Autodesk Inventor part; units mm, degrees
ref_plane "YZ Plane" through (0, 0, 0) normal (1, 0, 0) x (0, 1, 0)
ref_plane "XZ Plane" through (0, 0, 0) normal (0, 1, 0) x (-1, 0, 0)
ref_plane "XY Plane" through (0, 0, 0) normal (0, 0, 1) x (1, 0, 0)
sketch "Sketch2" plane through (0, 0, 0) normal (0, 0, 1) x (1, 0, 0)
  line L0 (0, 0) -> (48.55, 0)
  line L1 (48.55, 0) -> (48.55, -13)
  line L2 (48.55, -13) -> (44.55, -13)
  line L3 (44.55, -13) -> (44.55, -4)
  line L4 (44.55, -4) -> (38.45, -4)
  line L5 (38.45, -4) -> (38.45, -7)
  line L6 (38.45, -7) -> (0, -7)
  line L7 (0, -7) -> (0, 0)
  dimension "d0" = 48.55
  dimension "d1" = 4
  dimension "d2" = 6.1
  dimension "d3" = 13
  dimension "d4" = 4
  dimension "d5" = 7
revolve "Revolution1" add sketch "Sketch2" angle 360 about axis through (0, -7, 0) along (0, 1, 0)
fillet "Fillet1" radius 3 1 edges at (-48.55, 0, 0)
sketch "Sketch3" plane through (0, -7, 0) normal (0, -1, 0) x (1, 0, 0)
  circle A0 centre (0, -19.85) radius 17
  circle A1 centre (0, 0) radius 38.45
  circle A2 centre (17.1906, 9.925) radius 17
  circle A3 centre (-17.1906, 9.925) radius 17
  dimension "d8" = 34
  dimension "d11" = 360
  dimension "d15" = 19.85
extrude "Extrusion1" cut sketch "Sketch3" against normal blind 5.5 contours A0 | A2 | A3
sketch "Sketch5" plane through (0, -7, 0) normal (0, -1, 0) x (1, 0, 0)
  circle A0 centre (-25.9808, -15) radius 6.25
  line L0 (-25.9808, -15) -> (0, 0) construction
  line L1 (0, 0) -> (-9.9215, 0) construction
  dimension "d16" = 12.5
  dimension "d17" = 30
  dimension "d20" = 30
extrude "Extrusion2" cut sketch "Sketch5" against normal through all
properties part number "lid-proto-v2"
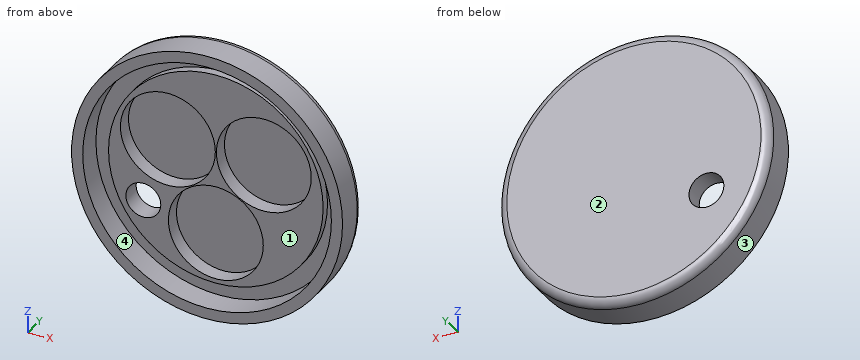
The listing builds one solid part. Answer for the finished solid, in the listing's coordinates (mm). Face numbers are marked on the shaded views. Coordinates: 2 decimals unless noted, no trailing zeros. Write each loop counter-clockwise with the first axis right and the second up, starting at its lowest first coordinate (ties: lowest second). Pieces come first, ordered by that corner, then holes. Notation, with made-up numbers: M 51.5,-17 L 94.5,-17 A25 cw 94.5,8 Z; hole C -34.5,-29.5 d6. An arc over 180 degrees is marked long. Write each question's results on one line, items separated by ' | '.
Item 1: The part is cut by section A-A on y = -10. Determine the outline of the cut face in (x, z).
Answer below:
outline: C 0,0 d97.1; hole C 0,0 d89.1
Item 2: For a pull along Z with two mould halves and no side action, classify the marked faces 1, 2, 3 and 4 as released by +Z, released by -Z, zero draft, split by the parting line, or undercut.
Answer below:
face 1: undercut | face 2: zero draft | face 3: split by the parting line | face 4: undercut
Item 3: Given P1, Ø3, axis at y = -8, z = -18, coming from the +X side; P2, Ø1.5, axis at y = -3.5, z = -33, coming from the +X side; P3, Ø5, axis at y = -8, z = -30, coming from the +X side, each flat-ended and moving along its own axis, determine where each tip first touches the part or whether it passes through.
Answer below:
P1: x = 45.66 | P2: x = 36.29 | P3: x = 40.01
Item 4: Consider probe 1 along Z at (x, y) = (0, -4.85); probe 2 along Y at (x, z) = (12, -25.5); probe 3 along X at (y, z) = (-6, 8). Determine where each line is inside the solid, lowest interval first. Write a range as [from, to].
Answer below:
probe 1: [-48.55, -44.55], [-38.45, -36.85], [-2.85, 38.45], [44.55, 48.55] | probe 2: [-1.5, 0] | probe 3: [-47.89, -43.83], [-37.61, -34.08], [-0.3, 0.3], [34.08, 37.61], [43.83, 47.89]
